Geometry check sheet. Reference: the model listing, model coordinates, mm. Face numbers are marked on the shaded views. A direction names the side the tool comes from. Coordinates: 2 decimals unless noted, no trailing zeros. Write each loop counter-clockwise with the first axis right and the second up, starting at its lowest first coordinate (ties: lowest second). Pieces come first, ordered by that corner, then holes. Notation, with made-up numbers: M 55.25,88.25 L 109.25,88.25 A25 cw 109.25,124.25 Z; hole C 23,45.25 d10. An arc over 180 degrees is marked long. Put each result on its own line as item: value. Start each with the question number.
1) Mould release check, pull along Z, two halves, no side actions. Record for the marked faces 6, 7 and 8: released by +Z, released by -Z, zero draft, split by the parting line, or undercut.
2) Set-up check for the marked faces 1, 2, 3, 4 and 5: record each of +Z, -Z, +X, -X, +Y, -Y from which the full face is reachable in a straight line by a thin tool's end or side.
3) Cross-section at C-C on z = 0. Record the cut outline in (x, y).
4) Scan lines: line 1 along Y through (x, z) = (20.5, 0); line 2 along Y through (x, z) = (1, 0); line 3 along Y through (x, z) = (-15.5, 2). Record each from-to range of solid material in increasing order.
5) Cross-section at D-D on z = 8.5. Record the cut outline in (x, y), plus the area to 3 significant figures.
6) Cross-section at B-B on x = -17.5. Record the cut outline in (y, z).
7) Cross-section at A-A on y = 0. Record the cut outline in (x, z), plus the area to 3 significant figures.
8) Gauge pin test, flat ends, axial feed: pin 1 (12 mm diameter, centred on x = 27, y = -5, fed in from -Z); pin 2 (1.5 mm diameter, centred on x = -1.5, z = -12.5, fed in from -Y); pin 3 (1.5 mm diameter, centred on y = 56, z = -2.5, fed in from +X); pin 4 (18 mm diameter, centred on x = -1, y = 44, fed in from -Z). Record the tip position at first contact, or that the pin passes through.
from build123d import *

# Parameters (mm, degrees)
SKETCH1_R           = 28
SKETCH1_R_2         = 16
BOSS_EXTRUDE1_DEPTH = 35
BOSS_EXTRUDE3_DEPTH = 30
BOSS_EXTRUDE4_DEPTH = 9
SKETCH5_R           = 25
SKETCH5_R_2         = 12.5
BOSS_EXTRUDE5_DEPTH = 30


with BuildPart() as part:
    # Sketch1 → Boss-Extrude1 (new, symmetric)
    with BuildSketch(Plane(origin=(0, 0, 0), x_dir=(0, 0, -1), z_dir=(1, 0, 0))):
        Circle(SKETCH1_R)
        Circle(SKETCH1_R_2, mode=Mode.SUBTRACT)
    extrude(amount=BOSS_EXTRUDE1_DEPTH, both=True)

    # Sketch2 → Boss-Extrude3 (add, symmetric)
    with BuildSketch(Plane(origin=(0, 0, 0), x_dir=(0, 0, -1), z_dir=(1, 0, 0))):
        with BuildLine():
            Line((-25, 40), (25, 40))
            Line((25, 40), (25, 12.609520213))
            ThreePointArc((25, 12.609520213), (0, 28), (-25, 12.609520213))
            Line((-25, 12.609520213), (-25, 40))
        make_face()
    extrude(amount=BOSS_EXTRUDE3_DEPTH, both=True)

    # Sketch3 → Boss-Extrude4 (add, symmetric)
    with BuildSketch(Plane(origin=(0, 0, 0), x_dir=(0, 0, -1), z_dir=(1, 0, 0))):
        with BuildLine():
            Line((-25, 40), (-25, 110))
            ThreePointArc((-25, 110), (0, 85), (25, 110))
            Line((25, 110), (25, 40))
            Line((25, 40), (-25, 40))
        make_face()
    extrude(amount=BOSS_EXTRUDE4_DEPTH, both=True)

    # Sketch5 → Boss-Extrude5 (add, symmetric)
    with BuildSketch(Plane(origin=(0, 0, 0), x_dir=(0, 0, -1), z_dir=(1, 0, 0))):
        with Locations((0, 110)):
            Circle(SKETCH5_R)
        with Locations((0, 110)):
            Circle(SKETCH5_R_2, mode=Mode.SUBTRACT)
    extrude(amount=BOSS_EXTRUDE5_DEPTH, both=True)


solid = part.part
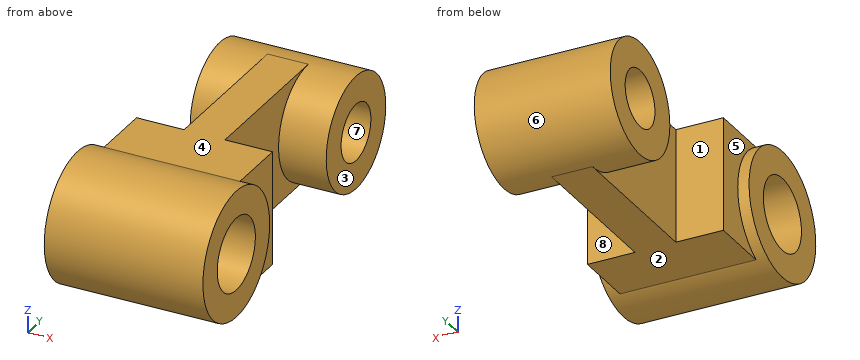
Answer key:
1. face 6: split by the parting line
1. face 7: undercut
1. face 8: zero draft
2. face 1: +Z, -Z, -X
2. face 2: -Z, +X, -X, +Y
2. face 3: +Z, -Z, +X, +Y
2. face 4: +Z, +X, -X, +Y
2. face 5: -X, +Y
3. outline: M -35,-28 L 35,-28 L 35,-16 L -35,-16 Z; M -35,16 L 35,16 L 35,28 L 30,28 L 30,40 L 9,40 L 9,85 L 30,85 L 30,97.5 L -30,97.5 L -30,85 L -9,85 L -9,40 L -30,40 L -30,28 L -35,28 Z; M -30,122.5 L 30,122.5 L 30,135 L -30,135 Z
4. line 1: y = -28 to -16, 16 to 40, 85 to 97.5, 122.5 to 135
4. line 2: y = -28 to -16, 16 to 97.5, 122.5 to 135
4. line 3: y = -27.93 to -15.87, 15.87 to 40, 85.08 to 97.66, 122.34 to 134.92
5. outline: M -35,-26.68 L 35,-26.68 L 35,-13.56 L -35,-13.56 Z; M -35,13.56 L 35,13.56 L 35,26.68 L 30,26.68 L 30,40 L 9,40 L 9,86.49 L 30,86.49 L 30,100.83 L -30,100.83 L -30,86.49 L -9,86.49 L -9,40 L -30,40 L -30,26.68 L -35,26.68 Z; M -30,119.17 L 30,119.17 L 30,133.51 L -30,133.51 Z
5. area: 5,190 mm²
6. outline: M 12.61,-25 L 40,-25 L 40,25 L 12.61,25 A28 ccw long Z; C 110,0 d50; hole C 0,0 d32; hole C 110,0 d25
7. outline: M -35,-28 L 35,-28 L 35,-16 L -35,-16 Z; M -35,16 L 35,16 L 35,28 L -35,28 Z
7. area: 1,680 mm²
8. pin 1: stops at z = -28
8. pin 2: stops at y = -25.42
8. pin 3: stops at x = 9
8. pin 4: stops at z = -25
